```python
from build123d import *

# Parameters (mm, degrees)
F0_W     = 50
F0_H     = 75
F0_R     = 2.5
F0_R_2   = 2
F0_H_2   = 30
F0_R_3   = 9.6
F1_DEPTH = 6
F2_DEPTH = 2
F3_DEPTH = 17
F0_R_4   = 8.5
F4_DEPTH = 11
F5_SIZE  = 1


with BuildPart() as f1:
    # F0 (on Top) → F1 (new body)
    with BuildSketch(Plane.XY):
        with Locations((25, 37.5)):
            Rectangle(F0_W, F0_H)
        with Locations((7, 7)):
            Circle(F0_R, mode=Mode.SUBTRACT)
        with Locations((43, 7)):
            Circle(F0_R, mode=Mode.SUBTRACT)
        Polygon((35.25, 5), (14.75, 5), (14.75, 13), (14.75, 53), (14.75, 61), (35.25, 61), (35.25, 53), (35.25, 13), align=None, mode=Mode.SUBTRACT)
        with Locations((7, 63)):
            Circle(F0_R, mode=Mode.SUBTRACT)
        with Locations((43, 63)):
            Circle(F0_R, mode=Mode.SUBTRACT)
        Polygon((14.75, 61), (14.75, 53), (24, 53), (24, 59), (26, 59), (26, 53), (35.25, 53), (35.25, 61), align=None)
        with Locations((20, 57)):
            Circle(F0_R_2, mode=Mode.SUBTRACT)
        with Locations((30, 57)):
            Circle(F0_R_2, mode=Mode.SUBTRACT)
        Polygon((14.75, 13), (14.75, 5), (35.25, 5), (35.25, 13), (26, 13), (26, 7), (24, 7), (24, 13), align=None)
        with Locations((20, 9)):
            Circle(F0_R_2, mode=Mode.SUBTRACT)
        with Locations((30, 9)):
            Circle(F0_R_2, mode=Mode.SUBTRACT)
        with Locations((25, 90)):
            Rectangle(F0_W, F0_H_2)
        with Locations((25, 88.0167)):
            Circle(F0_R_3, mode=Mode.SUBTRACT)
    extrude(amount=-F1_DEPTH)

    # F0 (on Top) → F2 (cut)
    with BuildSketch(Plane.XY):
        Polygon((14.75, 61), (14.75, 53), (24, 53), (24, 59), (26, 59), (26, 53), (35.25, 53), (35.25, 61), align=None)
        with Locations((20, 57)):
            Circle(F0_R_2, mode=Mode.SUBTRACT)
        with Locations((30, 57)):
            Circle(F0_R_2, mode=Mode.SUBTRACT)
        Polygon((14.75, 13), (14.75, 5), (35.25, 5), (35.25, 13), (26, 13), (26, 7), (24, 7), (24, 13), align=None)
        with Locations((20, 9)):
            Circle(F0_R_2, mode=Mode.SUBTRACT)
        with Locations((30, 9)):
            Circle(F0_R_2, mode=Mode.SUBTRACT)
    extrude(amount=-F2_DEPTH, mode=Mode.SUBTRACT)

    # F0 (on Top) → F3 (join)
    with BuildSketch(Plane.XY):
        with Locations((25, 90)):
            Rectangle(F0_W, F0_H_2)
        with Locations((25, 88.0167)):
            Circle(F0_R_3, mode=Mode.SUBTRACT)
    extrude(amount=F3_DEPTH)

    # F0 (on Top) → F4 (join)
    with BuildSketch(Plane.XY):
        with Locations((25, 88.0167)):
            Circle(F0_R_3)
        with Locations((25, 88.0167)):
            Circle(F0_R_4, mode=Mode.SUBTRACT)
    extrude(amount=F4_DEPTH)

    # F5
    f5_edges = [f1.edges().sort_by_distance(p)[0] for p in [
        (16.5, 88.0167, 11),
        (16.5, 88.0167, 0),
    ]]
    chamfer(f5_edges, length=F5_SIZE)


solid = f1.part
```
Source: CAD feature listing. Evaluate the final solid. Frame: model axes, mm. A direction names the side the tool comes from. Give positions to 0.01 mm unless a question says otherwise; leave off trailing zeros. Order: outer loops, then holes, each group sorted by start corner. A loop starts at its lowest first (then second) coordinate and runs counter-clockwise, first axis right, second up. Notation, with made-up numbers: (23.5, -9.5) -> (67.5, -9.5) arc R11 ccw to (67.5, 7.5) -> close; hole circle Ø9 at (-36.75, 41). An arc over 180 degrees is marked (long way). Use a Markdown table: item, result.
Q1. Section B-B (y = 17). Return the cut outline in (x, z).
A:
| item | result |
|---|---|
| outline | (0, -6) -> (14.75, -6) -> (14.75, 0) -> (0, 0) -> close; (35.25, -6) -> (50, -6) -> (50, 0) -> (35.25, 0) -> close |
Q2. Section C-C (y = 57). Return the cut outline in (x, z), and give its area (3 significant figures).
A:
| item | result |
|---|---|
| outline | (0, -6) -> (18, -6) -> (18, -2) -> (14.75, -2) -> (14.75, 0) -> (0, 0) -> close; (22, -6) -> (24, -6) -> (24, -2) -> (22, -2) -> close; (26, -6) -> (28, -6) -> (28, -2) -> (26, -2) -> close; (32, -6) -> (50, -6) -> (50, 0) -> (35.25, 0) -> (35.25, -2) -> (32, -2) -> close |
| area | 219 mm^2 |
Q3. Section A-A (x = 7). Return the cut outline in (y, z), and give its area (3 significant figures).
A:
| item | result |
|---|---|
| outline | (0, -6) -> (4.5, -6) -> (4.5, 0) -> (0, 0) -> close; (9.5, -6) -> (60.5, -6) -> (60.5, 0) -> (9.5, 0) -> close; (65.5, -6) -> (105, -6) -> (105, 17) -> (75, 17) -> (75, 0) -> (65.5, 0) -> close |
| area | 1,080 mm^2 |
Q4. First-contact query: P1, Ø15.5, axis at x = 28.5, y = 91.5, coming from the +Z side; P2, Ø1, axis at x = 29, z = 14, coming from the -Y side; P3, Ø4.5, axis at x = 20, y = 9, coming from the +Z side; P4, Ø1, axis at x = 34, y = 62, coming from the +Z side. Flat tips, straight axial feed; report the tip coordinate or a pass-through.
A:
| item | result |
|---|---|
| P1 | z = 17 |
| P2 | y = 75 |
| P3 | z = -2 |
| P4 | z = 0 |
Q5. Pull-direction query (X, two-part tool) for faces 1 (the face through (50, 75, -2)), 2 (the face through (25, 105, 5)), 3 (the face through (35.25, 33, -3)); classes: +X half, -X half, draft (parallel to the pull), parting line (faces both ways), or undercut.
A:
| item | result |
|---|---|
| face 1 | +X half |
| face 2 | draft |
| face 3 | undercut |
Q6. Section D-D (x = 25). State how many separate pieces and enclosed holes the cut face has, and give its area (3 significant figures).
A:
| item | result |
|---|---|
| separate pieces | 3 |
| enclosed holes | 0 |
| area | 401 mm^2 |
Q7. Material intervals for line 1 (Y direction, x = 7, z = -3.7); line 2 (Y direction, x = 30, z = -4.5); line 3 (Z direction, x = 2.5, y = 74), sorted ascending. Write a range as [from, to].
A:
| item | result |
|---|---|
| line 1 | [0, 4.5], [9.5, 60.5], [65.5, 105] |
| line 2 | [0, 7], [11, 13], [53, 55], [59, 79.82], [96.21, 105] |
| line 3 | [-6, 0] |
Q8. Access query for faces 4 (the face through (19, 53, -4)), 5 (the face through (25, 61, -1)), 6 (the face through (22.919, 78.645, -3.042)), 7 (the face through (36, 38, 0)). Directions: +Z, -Z, +X, -X, +Y, -Y. A direction counts if a zero-diameter tool reaches every point of the face in a straight line with its end or side. Return the directions, or none.
A:
| item | result |
|---|---|
| face 4 | +Z, -Z |
| face 5 | +Z |
| face 6 | -Z |
| face 7 | +Z, +X, -X, -Y |
